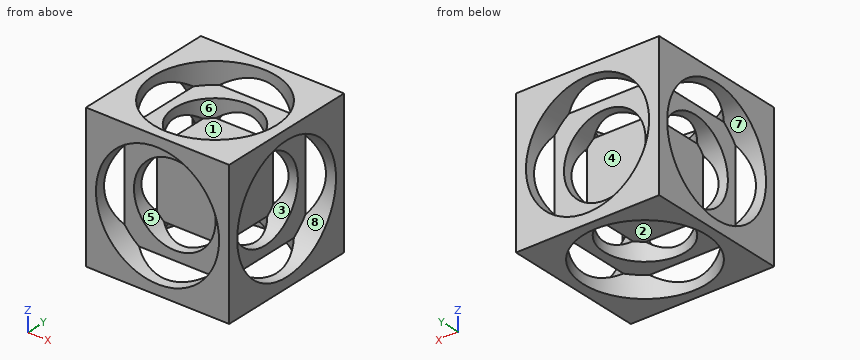
from build123d import *

# Parameters (mm, degrees)
F15_W     = 127
F15_H     = 127
F16_DEPTH = 127
F0_R      = 54.61
F17_DEPTH = 19.05
F18_R     = 54.61
F1_DEPTH  = 19.05
F19_R     = 54.61
F2_DEPTH  = 19.05
F3_R      = 54.61
F4_DEPTH  = 19.05
F20_R     = 54.61
F5_DEPTH  = 19.05
F6_R      = 54.61
F21_DEPTH = 19.05
F22_R     = 36.195
F7_DEPTH  = 15.875
F8_R      = 36.195
F9_DEPTH  = 15.875
F23_R     = 36.195
F10_DEPTH = 15.875
F11_R     = 36.195
F24_DEPTH = 15.875
F25_R     = 36.195
F12_DEPTH = 15.875
F13_R     = 36.195
F14_DEPTH = 15.875


with BuildPart() as f16:
    # F15 (on Top) → F16 (new body)
    with BuildSketch(Plane.XY):
        Rectangle(F15_W, F15_H)
    extrude(amount=F16_DEPTH)

    # F0 (on face) → F17 (cut)
    with BuildSketch(Plane.XY.offset(127)):
        Circle(F0_R)
    extrude(amount=-F17_DEPTH, mode=Mode.SUBTRACT)

    # F18 (on face) → F1 (cut)
    with BuildSketch(Plane.XZ.offset(63.5)):
        with Locations((0, 63.5)):
            Circle(F18_R)
    extrude(amount=-F1_DEPTH, mode=Mode.SUBTRACT)

    # F19 (on face) → F2 (cut)
    with BuildSketch(Plane(origin=(0, 63.5, 0), x_dir=(-1, 0, 0), z_dir=(0, 1, 0))):
        with Locations((0, 63.5)):
            Circle(F19_R)
    extrude(amount=-F2_DEPTH, mode=Mode.SUBTRACT)

    # F3 (on face) → F4 (cut)
    with BuildSketch(Plane.YZ.offset(63.5)):
        with Locations((0, 63.5)):
            Circle(F3_R)
    extrude(amount=-F4_DEPTH, mode=Mode.SUBTRACT)

    # F20 (on face) → F5 (cut)
    with BuildSketch(Plane(origin=(-63.5, 0, 0), x_dir=(0, -1, 0), z_dir=(-1, 0, 0))):
        with Locations((0, 63.5)):
            Circle(F20_R)
    extrude(amount=-F5_DEPTH, mode=Mode.SUBTRACT)

    # F6 (on face) → F21 (cut)
    with BuildSketch(Plane(origin=(0, 0, 0), x_dir=(1, 0, 0), z_dir=(0, 0, -1))):
        Circle(F6_R)
    extrude(amount=-F21_DEPTH, mode=Mode.SUBTRACT)

    # F22 (on face) → F7 (cut)
    with BuildSketch(Plane(origin=(0, 0, 19.05), x_dir=(1, 0, 0), z_dir=(0, 0, -1))):
        Circle(F22_R)
    extrude(amount=-F7_DEPTH, mode=Mode.SUBTRACT)

    # F8 (on face) → F9 (cut)
    with BuildSketch(Plane.XZ.offset(44.45)):
        with Locations((0, 63.5)):
            Circle(F8_R)
    extrude(amount=-F9_DEPTH, mode=Mode.SUBTRACT)

    # F23 (on face) → F10 (cut)
    with BuildSketch(Plane.YZ.offset(44.45)):
        with Locations((0, 63.5)):
            Circle(F23_R)
    extrude(amount=-F10_DEPTH, mode=Mode.SUBTRACT)

    # F11 (on face) → F24 (cut)
    with BuildSketch(Plane(origin=(-44.45, 0, 0), x_dir=(0, -1, 0), z_dir=(-1, 0, 0))):
        with Locations((0, 63.5)):
            Circle(F11_R)
    extrude(amount=-F24_DEPTH, mode=Mode.SUBTRACT)

    # F25 (on face) → F12 (cut)
    with BuildSketch(Plane(origin=(0, 44.45, 0), x_dir=(-1, 0, 0), z_dir=(0, 1, 0))):
        with Locations((0, 63.5)):
            Circle(F25_R)
    extrude(amount=-F12_DEPTH, mode=Mode.SUBTRACT)

    # F13 (on face) → F14 (cut)
    with BuildSketch(Plane.XY.offset(107.95)):
        Circle(F13_R)
    extrude(amount=-F14_DEPTH, mode=Mode.SUBTRACT)


solid = f16.part
Geometry: final body of the model. Coordinates: model frame, mm. Face numbers are marked on the shaded views. A direction names the side the tool comes from. Give positions to 0.01 mm unless a question says otherwise; leave off trailing zeros. Write each loop counter-clockwise with the first axis right and the second up, starting at its lowest first coordinate (ties: lowest second). Pieces come first, ordered by that corner, then holes. Notation, with made-up numbers: (87, 47) -> (122, 47) arc R12 ccw to (122, 58) -> close; hole circle Ø10 at (8.25, 79). An arc over 180 degrees is marked (long way). Answer in a Markdown table with one row per item.
(1) Section query C-C on x = -51.5. Return loops of the section in (y, z), then the cut area to 3 significant figures.
Answers below:
| item | result |
|---|---|
| outline | (-63.5, 0) -> (-18.17, 0) -> (-18.17, 12) arc R54.61 cw to (-51.5, 45.33) -> (-63.5, 45.33) -> close; (-63.5, 81.67) -> (-51.5, 81.67) arc R54.61 cw to (-18.17, 115) -> (-18.17, 127) -> (-63.5, 127) -> close; (18.17, 0) -> (63.5, 0) -> (63.5, 45.33) -> (51.5, 45.33) arc R54.61 cw to (18.17, 12) -> close; (18.17, 115) arc R54.61 cw to (51.5, 81.67) -> (63.5, 81.67) -> (63.5, 127) -> (18.17, 127) -> close |
| area | 5,320 mm^2 |
(2) Draft query along Z for the marked faces 1, 2 and 3. Return one class per face: +Z half, -Z half, draft (parallel to the pull), parting line (faces both ways), or undercut.
Answers below:
| item | result |
|---|---|
| face 1 | +Z half |
| face 2 | -Z half |
| face 3 | undercut |
(3) Set-up query: the marked faces 4, 5, 6, 7 and 8. Return all of +Z, -Z, +X, -X, +Y, -Y with unobstructed straight access to the full face (end or side cutting, diameter ignored); none if empty.
Answers below:
| item | result |
|---|---|
| face 4 | +Y |
| face 5 | -Y |
| face 6 | +Z |
| face 7 | -X |
| face 8 | +X |
(4) Section query D-D on z = 63.5. State how many separate pieces and enclosed holes the cut face has, then the cut area to 3 significant figures.
Answers below:
| item | result |
|---|---|
| separate pieces | 9 |
| enclosed holes | 0 |
| area | 3,850 mm^2 |
(5) Ray query, line 1 along X through (y, z) = (0, 25) (3 decimals); line 2 along X through (y, z) = (55.5, 62); line 3 along X through (y, z) = (-15, 53.5) (3 decimals). Return the intervals inside material, ascending. Write a range as [from, to].
Answers below:
| item | result |
|---|---|
| line 1 | [-44.45, -36.195], [36.195, 44.45] |
| line 2 | [-63.5, -54.59], [54.59, 63.5] |
| line 3 | [-28.575, 28.575] |
(6) Pin query (flat end, axial travel): pin 1 (12 mm diameter, centred on y = -7.5, z = 54.5, fed in from +X) (3 decimals); pin 2 (1 mm diameter, centred on x = -21, y = 38.5, fed in from -Z); pin 3 (5 mm diameter, centred on y = -20.5, z = 97.5, fed in from -X). Return the tip coordinate at first contact, or that it passes through.
Answers below:
| item | result |
|---|---|
| pin 1 | x = 28.575 |
| pin 2 | z = 19.05 |
| pin 3 | x = -44.45 |
(7) Section query B-B on z = 106. Return loops of the section in (x, y) (3 decimals).
Answers below:
| item | result |
|---|---|
| outline | (-63.5, -63.5) -> (-34.293, -63.5) -> (-34.293, -44.45) -> (34.293, -44.45) -> (34.293, -63.5) -> (63.5, -63.5) -> (63.5, -34.293) -> (44.45, -34.293) -> (44.45, 34.293) -> (63.5, 34.293) -> (63.5, 63.5) -> (34.293, 63.5) -> (34.293, 44.45) -> (-34.293, 44.45) -> (-34.293, 63.5) -> (-63.5, 63.5) -> (-63.5, 34.293) -> (-44.45, 34.293) -> (-44.45, -34.293) -> (-63.5, -34.293) -> close; hole circle Ø72.39 at (0, 0) |
(8) Section query A-A on y = -47. Return loops of the section in (x, z).
Answers below:
| item | result |
|---|---|
| outline | (-63.5, 0) -> (-27.81, 0) -> (-27.81, 16.5) arc R54.61 cw to (-47, 35.69) -> (-63.5, 35.69) -> close; (-63.5, 91.31) -> (-47, 91.31) arc R54.61 cw to (-27.81, 110.5) -> (-27.81, 127) -> (-63.5, 127) -> close; (27.81, 0) -> (63.5, 0) -> (63.5, 35.69) -> (47, 35.69) arc R54.61 cw to (27.81, 16.5) -> close; (27.81, 110.5) arc R54.61 cw to (47, 91.31) -> (63.5, 91.31) -> (63.5, 127) -> (27.81, 127) -> close |
